```python
from build123d import *

# Parameters (mm, degrees)
SKETCH1_R                = 1.651
BOSS_EXTRUDE2_DEPTH      = 5.3975
SKETCH4_W                = 37.082318314
SKETCH4_H                = 34.047903563
SKETCH4_W_2              = 37.024578492
SKETCH4_H_2              = 32.488734362
BOSS_EXTRUDE3_DEPTH      = 5.3975
SKETCH3_R                = 12.192
SKETCH3_R_2              = 12.1285
CUT_EXTRUDE2_DEPTH       = 101.410849545
SKETCH12_R               = 4
CUT_EXTRUDE10_DEPTH      = 83.312
SKETCH15_R               = 1.651
CUT_EXTRUDE17_DEPTH      = 83.312
SKETCH35_R               = 3.175
CUT_EXTRUDE37_DEPTH      = 103.378
CUT_EXTRUDE37_DEPTH_BACK = 48.768
SKETCH40_R               = 12.192
CUT_EXTRUDE43_DEPTH      = 25.4


with BuildPart() as part:
    # Sketch1 → Boss-Extrude2 (new body)
    with BuildSketch(Plane.XY):
        with BuildLine():
            Line((-66.623575407, 34.29), (-54.685575407, 34.29))
            Line((-54.685575407, 34.29), (-54.685575407, -34.29))
            Line((-54.685575407, -34.29), (-66.623575407, -34.29))
            ThreePointArc((-66.623575407, -34.29), (0, -74.93), (66.623575407, -34.29))
            Line((66.623575407, -34.29), (54.685575407, -34.29))
            Line((54.685575407, -34.29), (54.685575407, 34.29))
            Line((54.685575407, 34.29), (66.623575407, 34.29))
            ThreePointArc((66.623575407, 34.29), (0, 74.93), (-66.623575407, 34.29))
        make_face()
        with Locations((-45.466, 11.049)):
            Circle(SKETCH1_R, mode=Mode.SUBTRACT)
        with Locations((-20.067270032, 10.795)):
            Circle(SKETCH1_R, mode=Mode.SUBTRACT)
        with Locations(Location((-20.067270032, -10.795, 0), (0, 0, 180))):
            Circle(SKETCH1_R, mode=Mode.SUBTRACT)
        with Locations(Location((-45.466, -11.049, 0), (0, 0, 180))):
            Circle(SKETCH1_R, mode=Mode.SUBTRACT)
        with Locations((45.466, -11.049)):
            Circle(SKETCH1_R, mode=Mode.SUBTRACT)
        with Locations((20.067270032, -10.795)):
            Circle(SKETCH1_R, mode=Mode.SUBTRACT)
        with Locations(Location((20.067270032, 10.795, 0), (0, 0, 180))):
            Circle(SKETCH1_R, mode=Mode.SUBTRACT)
        with Locations(Location((45.466, 11.049, 0), (0, 0, 180))):
            Circle(SKETCH1_R, mode=Mode.SUBTRACT)
    extrude(amount=BOSS_EXTRUDE2_DEPTH)

    # Sketch4 → Boss-Extrude3 (add)
    with BuildSketch(Plane(origin=(0, 0, 0), x_dir=(-1, 0, 0), z_dir=(0, 0, -1))):
        with Locations((32.991199211, -1.421154886)):
            Rectangle(SKETCH4_W, SKETCH4_H)
        with Locations((-34.085074962, -0.641570285)):
            Rectangle(SKETCH4_W_2, SKETCH4_H_2)
    extrude(amount=-BOSS_EXTRUDE3_DEPTH)

    # Sketch3 → Cut-Extrude2 (cut, through all)
    with BuildSketch(Plane(origin=(0, 0, 0), x_dir=(-1, 0, 0), z_dir=(0, 0, -1))):
        Circle(SKETCH3_R)
        with Locations((-42.926, -42.926)):
            Circle(SKETCH3_R_2)
        with Locations((15.777608989, -58.882838371)):
            Circle(SKETCH3_R_2)
        with Locations(Location((15.777608989, 58.882838371, 0), (0, 0, 180))):
            Circle(SKETCH3_R_2)
        with Locations((-42.926, 42.926)):
            Circle(SKETCH3_R_2)
        with Locations((42.926, 42.926)):
            Circle(SKETCH3_R_2)
        with Locations((-15.777608989, 58.882838371)):
            Circle(SKETCH3_R_2)
        with Locations(Location((-15.777608989, -58.882838371, 0), (0, 0, 180))):
            Circle(SKETCH3_R_2)
        with Locations((42.926, -42.926)):
            Circle(SKETCH3_R_2)
    extrude(amount=-CUT_EXTRUDE2_DEPTH, mode=Mode.SUBTRACT)

    # Sketch12 → Cut-Extrude10 (cut)
    with BuildSketch(Plane(origin=(0, 0, 0), x_dir=(-1, 0, 0), z_dir=(0, 0, -1))):
        with Locations((25.937608989, 45.466)):
            Circle(SKETCH12_R)
        with Locations((25.937608989, -45.466)):
            Circle(SKETCH12_R)
        with Locations(Location((-25.937608989, 45.466, 0), (0, 0, 180))):
            Circle(SKETCH12_R)
        with Locations(Location((-25.937608989, -45.466, 0), (0, 0, 180))):
            Circle(SKETCH12_R)
    extrude(amount=-CUT_EXTRUDE10_DEPTH, mode=Mode.SUBTRACT)

    # Sketch15 → Cut-Extrude17 (cut)
    with BuildSketch(Plane(origin=(0, 0, 0), x_dir=(-1, 0, 0), z_dir=(0, 0, -1))):
        with Locations((0, 66.04)):
            Circle(SKETCH15_R)
        with Locations(Location((0, -66.04, 0), (0, 0, 180))):
            Circle(SKETCH15_R)
    extrude(amount=-CUT_EXTRUDE17_DEPTH, mode=Mode.SUBTRACT)

    # Sketch35 → Cut-Extrude37 (cut, two sides)
    with BuildSketch(Plane(origin=(-30.092005081, 4.08352975, -42.4815), x_dir=(1, 0, 0), z_dir=(0, 0, 1))) as cut_extrude37_sk:
        with Locations((-16.897994919, 21.31647025)):
            Circle(SKETCH35_R)
        with Locations((77.082005081, 21.31647025)):
            Circle(SKETCH35_R)
        with Locations((30.092005081, 21.31647025)):
            Circle(SKETCH35_R)
        with Locations((77.082005081, -29.48352975)):
            Circle(SKETCH35_R)
        with Locations((30.092005081, -29.48352975)):
            Circle(SKETCH35_R)
        with Locations((-16.897994919, -29.48352975)):
            Circle(SKETCH35_R)
    extrude(amount=CUT_EXTRUDE37_DEPTH, mode=Mode.SUBTRACT)
    extrude(cut_extrude37_sk.sketch, amount=-CUT_EXTRUDE37_DEPTH_BACK, mode=Mode.SUBTRACT)

    # Sketch40 → Cut-Extrude43 (cut)
    with BuildSketch(Plane(origin=(0, 0, 0), x_dir=(-1, 0, 0), z_dir=(0, 0, -1))):
        with Locations((-31.75, 0)):
            Circle(SKETCH40_R)
        with Locations((31.75, 0)):
            Circle(SKETCH40_R)
        with BuildLine():
            Line((12.7, -20.32), (-12.7, -20.32))
            ThreePointArc((-12.7, -20.32), (-19.05, -13.97), (-12.7, -7.62))
            ThreePointArc((-12.7, -7.62), (0, -13.723935563), (12.7, -7.62))
            ThreePointArc((12.7, -7.62), (19.05, -13.97), (12.7, -20.32))
        make_face()
        with BuildLine():
            Line((12.7, 20.32), (-12.7, 20.32))
            ThreePointArc((-12.7, 20.32), (-19.05, 13.97), (-12.7, 7.62))
            ThreePointArc((-12.7, 7.62), (0, 13.723935563), (12.7, 7.62))
            ThreePointArc((12.7, 7.62), (19.05, 13.97), (12.7, 20.32))
        make_face()
    extrude(amount=-CUT_EXTRUDE43_DEPTH, mode=Mode.SUBTRACT)


solid = part.part
```
Model file for the job. Use its own axes, mm. A direction names the side the tool comes from. Give positions to 0.01 mm unless a question says otherwise; leave off trailing zeros. Order: outer loops, then holes, each group sorted by start corner. A loop starts at its lowest first (then second) coordinate and runs counter-clockwise, first axis right, second up.
1) Saw through at A-A, the plane x = 0. Count the separate pieces of the cut face and the enclosed holes in it, then the cut area to 3 significant figures.
2) Mould opens along X. For faces 1 (the cylindrical face through (43.93, 0.54, 2.66)), 2 (the cylindrical face through (1.15, 74.92, 2.66)), 3 (the flat face through (61, 34.29, 3)) say: +X half, -X half, draft (parallel to the pull), parting line (faces both ways), or undercut.
3) Pin check, flat tips, straight feed: pin 1 (7.5 mm diameter, centred on x = -46.99, y = -25.4, fed in from -Z); pin 2 (1.6 mm diameter, centred on x = 61.5, z = 2.5, fed in from -Y); pin 3 (1.6 mm diameter, centred on y = 14, z = 1.5, fed in from +X). Stop position of each tip, or through.
4) Saw through at D-D, the plane x = 46.99. Write the cut outline in (y, z) (1 decimal).
5) Wall check: probe 1 along X at (y, z) = (25.4, 3.8) (3 decimals); probe 2 along X at (y, z) = (44, 0.3); probe 3 along X at (y, z) = (-33, 0.55). Give the ranges that are in metal, low to high.
6) 3-axis set-ups, long thin cutter, end or side, ignore diameter. For faces 4 (the flat face through (0, -20.32, 3)), 5 (the flat face through (-16, 1, 0)), 6 (the flat face through (61, -34.29, 3)): which of +Z, -Z, +X, -X, +Y, -Y reach the whole face in a straight line?
7) Saw through at B-B, the plane y = 0. Write the cut outline in (x, z).
8) Saw through at C-C, the plane y = 51.5. Write the cut outline in (x, z).
Computed:
1. separate pieces: 8
1. enclosed holes: 0
1. area: 502 mm2
2. face 1: undercut
2. face 2: parting line
2. face 3: draft
3. pin 1: stops at z = 0
3. pin 2: stops at y = -43.93
3. pin 3: stops at x = 54.69
4. outline: (-58.4, 0) - (-54.4, 0) - (-54.4, 5.4) - (-58.4, 5.4) - close; (-31.5, 0) - (-28.6, 0) - (-28.6, 5.4) - (-31.5, 5.4) - close; (-22.2, 0) - (22.2, 0) - (22.2, 5.4) - (-22.2, 5.4) - close; (28.6, 0) - (31.5, 0) - (31.5, 5.4) - (28.6, 5.4) - close; (54.4, 0) - (58.4, 0) - (58.4, 5.4) - (54.4, 5.4) - close
5. probe 1: x = -54.686 to -50.165, -43.815 to -3.175, 3.175 to 43.815, 50.165 to 54.686
5. probe 2: x = -60.65 to -55.01, -30.85 to -29.66, -22.22 to 22.22, 29.66 to 30.85, 55.01 to 60.65
5. probe 3: x = -54.69 to -49.9, -35.96 to 35.96, 49.9 to 54.69
6. face 4: +Z, -Z
6. face 5: -Z, +X, -X, +Y, -Y
6. face 6: +Z, -Z, +X
7. outline: (-54.69, 0) - (-43.94, 0) - (-43.94, 5.4) - (-54.69, 5.4) - close; (-19.56, 0) - (-12.19, 0) - (-12.19, 5.4) - (-19.56, 5.4) - close; (12.19, 0) - (19.56, 0) - (19.56, 5.4) - (12.19, 5.4) - close; (43.94, 0) - (54.69, 0) - (54.69, 5.4) - (43.94, 5.4) - close
8. outline: (-54.43, 0) - (-51.5, 0) - (-51.5, 5.4) - (-54.43, 5.4) - close; (-34.35, 0) - (-25.4, 0) - (-25.4, 5.4) - (-34.35, 5.4) - close; (-6.16, 0) - (6.16, 0) - (6.16, 5.4) - (-6.16, 5.4) - close; (25.4, 0) - (34.35, 0) - (34.35, 5.4) - (25.4, 5.4) - close; (51.5, 0) - (54.43, 0) - (54.43, 5.4) - (51.5, 5.4) - close
